Geometry check sheet. Reference: drawing and pictorial views, mm from the part's lowest x, y, z. A direction names the side the tool comes from. Give positions to 0.01 mm unless a question says otherwise; leave off trailing zeros. Write each loop counter-clockwise with the first axis right and the second up, starting at its lowest first coordinate (ties: lowest second). Pieces come first, ordered by that corner, then holes. Notation, with made-up numbers: M -40,43.5 L -3,43.5 A21 cw -3,55.5 Z; hole C -11,-6 d6. An arc over 180 degrees is marked long. Answer as a JSON object with one key per item and string values.
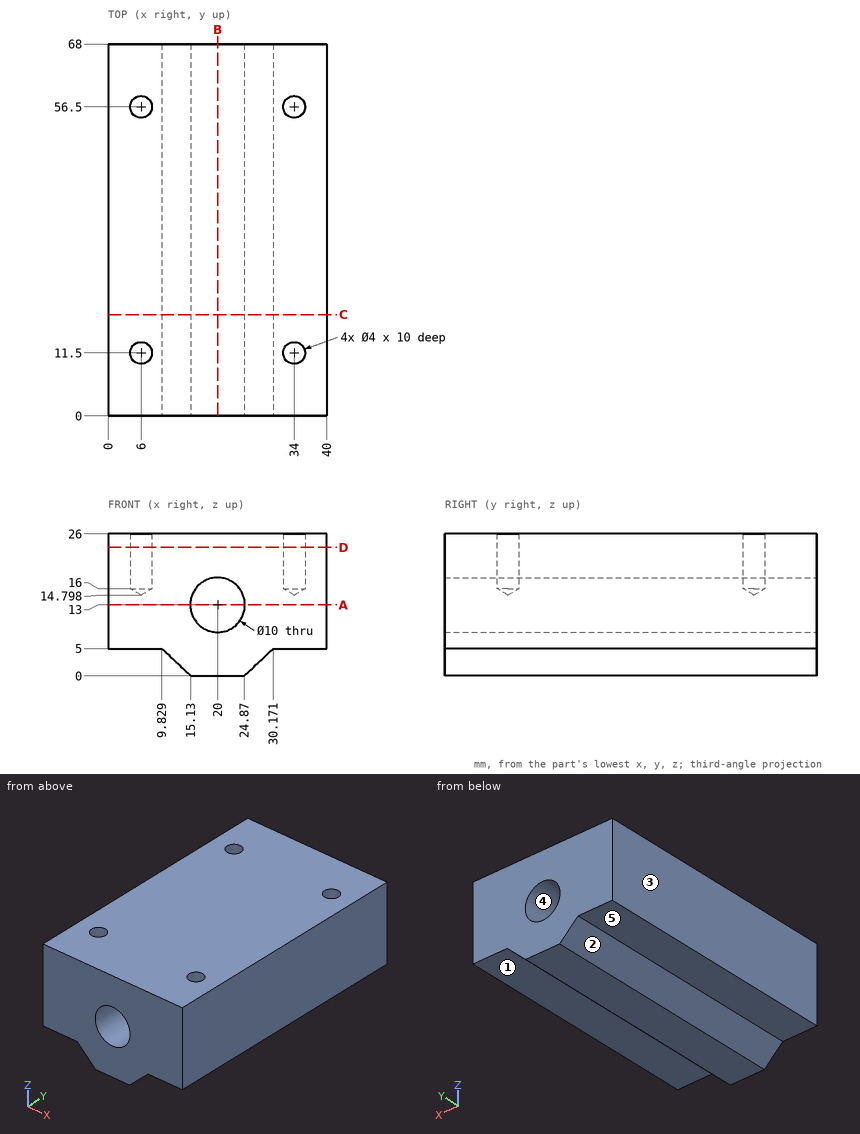
1) Access from +Z, -Z, +X, -X, +Y, -Y to the whole of each face (thin tool, end or side, straight path). Record for the marked faces 1 and 2.
Completed:
{"face 1": "-Z, +X, +Y, -Y", "face 2": "-Z, -X, +Y, -Y"}
2) Go/stop test with flat-tipped pins: pin 1 (3 mm diameter, centred on x = 34, y = 56.5, fed in from +Z); pin 2 (3 mm diameter, centred on x = 36, y = 28.5, fed in from -Z). Record where each tip stops, or that it passes through.
Completed:
{"pin 1": "stops at z = 15.7", "pin 2": "stops at z = 5"}
3) Release check for a two-part mould opening along X. For the marked faces 3, 4 and 5 record: pulls with the +X half, pulls with the -X half, needs draft (parallel to the pull), parting line crosses it, or undercut.
Completed:
{"face 3": "pulls with the -X half", "face 4": "undercut", "face 5": "needs draft"}
4) Section check C-C on y = 18.5. Record the boundary of the cut face in (x, z), and give its area (3 significant figures).
Completed:
{"outline": "M 0,5 L 9.83,5 L 15.13,0 L 24.87,0 L 30.17,5 L 40,5 L 40,26 L 0,26 Z; hole C 20,13 d10", "area": "837 mm2"}
5) Section check D-D on z = 23.5. Record the boundary of the cut face in (x, y).
Completed:
{"outline": "M 0,0 L 40,0 L 40,68 L 0,68 Z; hole C 6,11.5 d4; hole C 6,56.5 d4; hole C 34,11.5 d4; hole C 34,56.5 d4"}
6) Section check A-A on z = 13. Record the boundary of the cut face in (x, y).
Completed:
{"outline": "M 0,0 L 15,0 L 15,68 L 0,68 Z; M 25,0 L 40,0 L 40,68 L 25,68 Z"}
7) Section check B-B on x = 20. Record the boundary of the cut face in (y, z).
Completed:
{"outline": "M 0,0 L 68,0 L 68,8 L 0,8 Z; M 0,18 L 68,18 L 68,26 L 0,26 Z"}
8) Thickness scan on L1, parallel to X at y = 56.5, z = 23.25; L2, parallel to Z at x = 2, y = 22; L3, parallel to Z at x = 18, y = 21.5. Record the ranges inside material, lowest first.
Completed:
{"L1": "x = 0 to 4, 8 to 32, 36 to 40", "L2": "z = 5 to 26", "L3": "z = 0 to 8.42, 17.58 to 26"}
